Read the model definition and answer for the solid it produces. Units are mm, in the model's axes. Face numbers are marked on the shaded views. A direction names the side the tool comes from. Give positions to 0.01 mm unless a question says otherwise; leave off trailing zeros. Write each loop counter-clockwise with the first axis right and the second up, starting at its lowest first coordinate (ties: lowest second). Pieces come first, ordered by that corner, then holes. Notation, with made-up numbers: M -37,-32.5 L -25,-32.5 A24 cw -25,-1.5 Z; hole C -15.5,10.25 d8. An arc over 180 degrees is marked long. Use a Markdown table: item, result. Add a question column.
Item 1: For the marked faces 1, 2, 3 and 4, determine the directions among +Z, -Z, +X, -X, +Y, -Y from which every point of the face is accessible in a straight line to the end or side of a thin tool.
Item 2: A cutting plane is placed at B-B on z = 74. Determine the outline of the cut face in (x, y), then the cut area to 3 significant figures.
Item 3: Given P1, Ø3, axis at y = -3, z = 90.5, coming from the -X side; P2, Ø2, axis at y = 19, z = 56.5, coming from the -X side; P3, Ø10, axis at y = -20.5, z = 53.5, coming from the +X side, each flat-ended and moving along its own axis, determine where each tip first touches the part or whether it passes through.
Item 4: A cutting plane is placed at A-A on x = 0. Determine the outline of the cut face in (y, z).
Item 5: Consider probe 1 along Z at (x, y) = (1, 22); probe 2 along X at (y, z) = (-20, 24.5); probe 3 along Y at (x, z) = (-3.5, 102.5). Determine where each line is inside the solid, lowest interval first. Write a range as [from, to].
Item 6: The mould has two halves that part along Y. Classify the marked faces 5, 6 and 7: pulls with the +Y half, pulls with the -Y half, needs draft (parallel to the pull), parting line crosses it, or undercut.
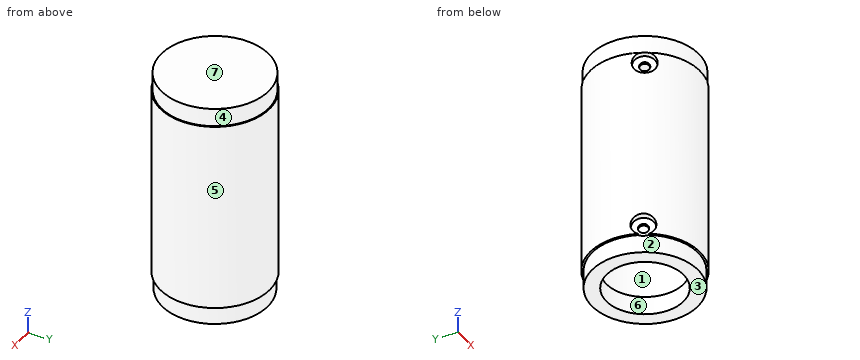
from build123d import *

# Parameters (mm, degrees)
SKETCH1_R                               = 30
SKETCH1_R_2                             = 25
BOSS_EXTRUDE1_DEPTH                     = 125
SKETCH2_R                               = 25
SKETCH2_R_2                             = 21.1
BOSS_EXTRUDE2_DEPTH                     = 10
SKETCH3_R                               = 25
BOSS_EXTRUDE3_DEPTH                     = 10
SKETCH11_R                              = 30
SKETCH11_R_2                            = 28.945980101
CUT_EXTRUDE2_DEPTH                      = 10
CUT_EXTRUDE3_START                      = -10
SKETCH12_R                              = 30
SKETCH12_R_2                            = 29.420954363
CUT_EXTRUDE3_DEPTH                      = 10
CBORE_START                             = -30.0000001
CBORE_FOR_M5_HEX_HEAD_BOLT2_OUTLINE_R   = 6.12
CBORE_FOR_M5_HEX_HEAD_BOLT2_DEPTH       = 3.5800001
CBORE_START_2                           = -26.42
CBORE_FOR_M5_HEX_HEAD_BOLT2_2_OUTLINE_R = 2.65
CBORE_FOR_M5_HEX_HEAD_BOLT2_2_DEPTH     = 1.560846858
CBORE_FOR_M5_HEX_HEAD_BOLT2_3_OUTLINE_R = 6.12
CBORE_FOR_M5_HEX_HEAD_BOLT2_3_DEPTH     = 3.5800001
CBORE_FOR_M5_HEX_HEAD_BOLT2_4_OUTLINE_R = 2.65
CBORE_FOR_M5_HEX_HEAD_BOLT2_4_DEPTH     = 1.560846858


# Read off the part's stored shape, not the designer's step: CBORE for M5 Hex Head Bolt2
with BuildPart() as part:
    # Sketch1 → Boss-Extrude1 (new body)
    with BuildSketch(Plane.XY):
        Circle(SKETCH1_R)
        Circle(SKETCH1_R_2, mode=Mode.SUBTRACT)
    extrude(amount=BOSS_EXTRUDE1_DEPTH)

    # Sketch2 → Boss-Extrude2 (add)
    with BuildSketch(Plane.XY):
        Circle(SKETCH2_R)
        Circle(SKETCH2_R_2, mode=Mode.SUBTRACT)
    extrude(amount=BOSS_EXTRUDE2_DEPTH)

    # Sketch3 → Boss-Extrude3 (add)
    with BuildSketch(Plane.XY.offset(115)):
        Circle(SKETCH3_R)
    extrude(amount=BOSS_EXTRUDE3_DEPTH)

    # Sketch11 → Cut-Extrude2 (cut)
    with BuildSketch(Plane(origin=(0, 0, 0), x_dir=(-1, 0, 0), z_dir=(0, 0, -1))):
        Circle(SKETCH11_R)
        Circle(SKETCH11_R_2, mode=Mode.SUBTRACT)
    extrude(amount=-CUT_EXTRUDE2_DEPTH, mode=Mode.SUBTRACT)

    # Sketch12 → Cut-Extrude3 (cut)
    with BuildSketch(Plane.XY.offset(125).offset(CUT_EXTRUDE3_START)):
        with Locations(Location((0, 0, 0), (0, 0, 180))):
            Circle(SKETCH12_R)
        Circle(SKETCH12_R_2, mode=Mode.SUBTRACT)
    extrude(amount=CUT_EXTRUDE3_DEPTH, mode=Mode.SUBTRACT)

    # CBORE for M5 Hex Head Bolt2 outline → CBORE for M5 Hex Head Bolt2 (cut)
    with BuildSketch(Plane(origin=(0, 0, 0), x_dir=(0.48168847359227474, -0.8763425211687177, 0), z_dir=(0.8763425211687177, 0.48168847359227485, 0)).offset(CBORE_START)):
        with Locations((0, -15.551111343)):
            Circle(CBORE_FOR_M5_HEX_HEAD_BOLT2_OUTLINE_R)
    extrude(amount=CBORE_FOR_M5_HEX_HEAD_BOLT2_DEPTH, mode=Mode.SUBTRACT)

    # CBORE for M5 Hex Head Bolt2 2 outline → CBORE for M5 Hex Head Bolt2 2 (cut)
    with BuildSketch(Plane(origin=(0, 0, 0), x_dir=(0.48168847359227474, -0.8763425211687177, 0), z_dir=(0.8763425211687177, 0.48168847359227485, 0)).offset(CBORE_START_2)):
        with Locations((0, -15.551111343)):
            Circle(CBORE_FOR_M5_HEX_HEAD_BOLT2_2_OUTLINE_R)
    extrude(amount=CBORE_FOR_M5_HEX_HEAD_BOLT2_2_DEPTH, mode=Mode.SUBTRACT)

    # CBORE for M5 Hex Head Bolt2 3 outline → CBORE for M5 Hex Head Bolt2 3 (cut)
    with BuildSketch(Plane(origin=(0, 0, 0), x_dir=(0.49930336052922, -0.8664272353546071, 0), z_dir=(0.8664272353546071, 0.49930336052922003, 0)).offset(CBORE_START)):
        with Locations((0, -109.335103389)):
            Circle(CBORE_FOR_M5_HEX_HEAD_BOLT2_3_OUTLINE_R)
    extrude(amount=CBORE_FOR_M5_HEX_HEAD_BOLT2_3_DEPTH, mode=Mode.SUBTRACT)

    # CBORE for M5 Hex Head Bolt2 4 outline → CBORE for M5 Hex Head Bolt2 4 (cut)
    with BuildSketch(Plane(origin=(0, 0, 0), x_dir=(0.49930336052922, -0.8664272353546071, 0), z_dir=(0.8664272353546071, 0.49930336052922003, 0)).offset(CBORE_START_2)):
        with Locations((0, -109.335103389)):
            Circle(CBORE_FOR_M5_HEX_HEAD_BOLT2_4_OUTLINE_R)
    extrude(amount=CBORE_FOR_M5_HEX_HEAD_BOLT2_4_DEPTH, mode=Mode.SUBTRACT)


solid = part.part
Filled in:
| question | item | result |
|---|---|---|
| 1 | face 1 | none |
| 1 | face 2 | -Z |
| 1 | face 3 | -Z, +X, -X, +Y, -Y |
| 1 | face 4 | +Z |
| 2 | outline | C 0,0 d60; hole C 0,0 d50 |
| 2 | area | 864 mm² |
| 3 | P1 | x = -29.96 |
| 3 | P2 | x = -24 |
| 3 | P3 | x = 25.69 |
| 4 | outline | M -30,10 L -28.95,10 L -28.95,0 L -21.1,0 L -21.1,10 L -25,10 L -25,115 L 25,115 L 25,10 L 21.1,10 L 21.1,0 L 28.95,0 L 28.95,10 L 30,10 L 30,115 L 29.42,115 L 29.42,125 L -29.42,125 L -29.42,115 L -30,115 Z |
| 5 | probe 1 | [0, 10], [115, 125] |
| 5 | probe 2 | [-22.36, -15], [15, 22.36] |
| 5 | probe 3 | [-29.8, -24.75], [24.75, 29.8] |
| 6 | face 5 | parting line crosses it |
| 6 | face 6 | undercut |
| 6 | face 7 | needs draft |
